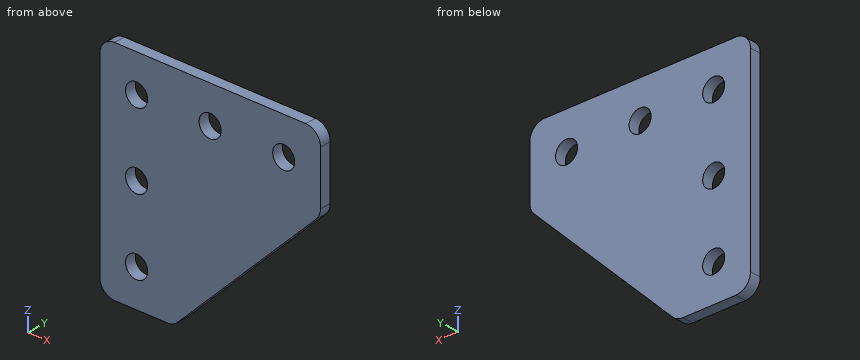
```python
from build123d import *

# Parameters (mm, degrees)
SKETCH_2_R      = 1.5
EXTRUDE_1_DEPTH = 1.5
FILLET_1_R      = 2


with BuildPart() as part:
    # ｽｹｯﾁ2 → ﾎﾞｽ - 押し出し1 (new body)
    with BuildSketch(Plane(origin=(0, 0, 0), x_dir=(1, 0, 0), z_dir=(0, 1, 0))):
        Polygon((0, 0), (30, 0), (30, 10), (10, 30), (0, 30), align=None)
        with Locations(Location((5, 5, 0), (0, 0, 270))):
            Circle(SKETCH_2_R, mode=Mode.SUBTRACT)
        with Locations(Location((25, 5, 0), (0, 0, 270))):
            Circle(SKETCH_2_R, mode=Mode.SUBTRACT)
        with Locations(Location((5, 25, 0), (0, 0, 90))):
            Circle(SKETCH_2_R, mode=Mode.SUBTRACT)
        with Locations(Location((15, 5, 0), (0, 0, 270))):
            Circle(SKETCH_2_R, mode=Mode.SUBTRACT)
        with Locations(Location((5, 15, 0), (0, 0, 270))):
            Circle(SKETCH_2_R, mode=Mode.SUBTRACT)
    extrude(amount=EXTRUDE_1_DEPTH)

    # ﾌｨﾚｯﾄ1
    fillet_1_edges = [part.edges().sort_by_distance(p)[0] for p in [
        (0, 0.75, -30),
        (10, 0.75, -30),
        (30, 0.75, -10),
        (30, 0.75, 0),
        (0, 0.75, 0),
    ]]
    fillet(fillet_1_edges, radius=FILLET_1_R)


solid = part.part
```
Geometry: final body of the model. Coordinates: model frame, mm. Round coordinates to 2 decimals unless told otherwise and drop trailing zeros. Write each loop counter-clockwise with the first axis right and the second up, starting at its lowest first coordinate (ties: lowest second). Pieces come first, ordered by that corner, then holes. Notation, with made-up numbers: M -38.5,69.5 L 13.5,69.5 A36 ccw 13.5,107.5 Z; hole C 36,-9 d4. An arc over 180 degrees is marked long. Answer in a Markdown table with one row per item. Add a question column.
(1) Cut plane A-A, the plane x = 25. Return the cut outline in (y, z), then the cut area to 3 significant figures.
(2) Ray query, L1, parallel to X at y = 0.9, z = -5; L2, parallel to Z at x = 5.5, y = 1.2; L3, parallel to X at y = 1, z = -14. Return the intervals inside material, ascending.
(3) Cut plane C-C, the plane z = -15. Return the cut outline in (x, y), then the cut area to 3 significant figures.
(4) Cut plane B-B, the plane y = 0.5. Return the cut outline in (x, z).
(5) Cut plane D-D, the plane z = -5. Return the cut outline in (x, y), then the cut area to 3 significant figures.
(6) Contact query for a flat-ended pin moving along its axis: pin 1 (2.5 mm diameter, centred on x = 25, z = -5, fed in from -Y). Output: stop coordinate, or through.
Established:
| question | item | result |
|---|---|---|
| 1 | outline | M 0,-15 L 1.5,-15 L 1.5,-6.5 L 0,-6.5 Z; M 0,-3.5 L 1.5,-3.5 L 1.5,0 L 0,0 Z |
| 1 | area | 18.0 mm² |
| 2 | L1 | 0 to 3.5, 6.5 to 13.5, 16.5 to 23.5, 26.5 to 30 |
| 2 | L2 | -30 to -26.41, -23.59 to -16.41, -13.59 to -6.41, -3.59 to 0 |
| 2 | L3 | 0 to 3.88, 6.12 to 26 |
| 3 | outline | M 0,0 L 3.5,0 L 3.5,1.5 L 0,1.5 Z; M 6.5,0 L 25,0 L 25,1.5 L 6.5,1.5 Z |
| 3 | area | 33.0 mm² |
| 4 | outline | M 0,-28 A2 ccw 2,-30 L 9.17,-30 A2 ccw 10.59,-29.41 L 29.41,-10.59 A2 ccw 30,-9.17 L 30,-2 A2 ccw 28,0 L 2,0 A2 ccw 0,-2 Z; hole C 5,-25 d3; hole C 5,-15 d3; hole C 5,-5 d3; hole C 15,-5 d3; hole C 25,-5 d3 |
| 5 | outline | M 0,0 L 3.5,0 L 3.5,1.5 L 0,1.5 Z; M 6.5,0 L 13.5,0 L 13.5,1.5 L 6.5,1.5 Z; M 16.5,0 L 23.5,0 L 23.5,1.5 L 16.5,1.5 Z; M 26.5,0 L 30,0 L 30,1.5 L 26.5,1.5 Z |
| 5 | area | 31.5 mm² |
| 6 | pin 1 | through |
